```python
from build123d import *

# Parameters (mm, degrees)
SKETCH1_W               = 5.08
SKETCH1_H               = 11.684
BOSS_EXTRUDE1_DEPTH     = 8.89
SKETCH2_R               = 4.318
CUT_EXTRUDE1_DEPTH      = 8.89
BOSS_EXTRUDE4_START     = -8.89
BOSS_EXTRUDE4_DEPTH     = 8.89
BOSS_EXTRUDE5_START     = -8.89
BOSS_EXTRUDE5_DEPTH     = 8.89
SKETCH9_W               = 3.302
SKETCH9_H               = 8.128
CUT_EXTRUDE4_DEPTH      = 8.89
CUT_EXTRUDE5_REACH      = 23.984
CUT_EXTRUDE5_END_RADIUS = 4.318
SKETCH10_R              = 1.905
SKETCH11_W              = 2.413
SKETCH11_H              = 8.89
SKETCH11_W_2            = 1.778
BOSS_EXTRUDE6_DEPTH     = 17.78
CUT_EXTRUDE6_REACH      = 27.049
SKETCH12_R              = 1.905
CUT_EXTRUDE7_START      = -8.89
CUT_EXTRUDE7_DEPTH      = 8.89
FILLET3_R               = 0.635
FILLET4_R               = 1.905


with BuildPart() as part:
    # Sketch1 → Boss-Extrude1 (new body)
    with BuildSketch(Plane(origin=(0, 0, 0), x_dir=(1, 0, 0), z_dir=(0, 1, 0))):
        Rectangle(SKETCH1_W, SKETCH1_H)
    extrude(amount=BOSS_EXTRUDE1_DEPTH)

    # Sketch2 → Cut-Extrude1 (cut)
    with BuildSketch(Plane(origin=(0, 8.89, 0), x_dir=(1, 0, 0), z_dir=(0, 1, 0))):
        with Locations((-5.08, 0)):
            Circle(SKETCH2_R)
    extrude(amount=-CUT_EXTRUDE1_DEPTH, mode=Mode.SUBTRACT)

    # Sketch7 → Boss-Extrude4 (add)
    with BuildSketch(Plane.XZ.offset(BOSS_EXTRUDE4_START)):
        with BuildLine():
            Line((-2.54, 3.49192268), (-2.54, 5.842))
            ThreePointArc((-2.54, 5.842), (-11.450287592, 0), (-2.54, -5.842))
            Line((-2.54, -5.842), (-2.54, -3.49192268))
            ThreePointArc((-2.54, -3.49192268), (-9.398, 0), (-2.54, 3.49192268))
        make_face()
    extrude(amount=BOSS_EXTRUDE4_DEPTH)

    # Sketch8 → Boss-Extrude5 (add)
    with BuildSketch(Plane.XZ.offset(BOSS_EXTRUDE5_START)):
        with BuildLine():
            Line((-7.894132015, 5.715), (-16.530287592, 5.715))
            Line((-16.530287592, 5.715), (-16.530287592, -5.715))
            Line((-16.530287592, -5.715), (-7.894132015, -5.715))
            ThreePointArc((-7.894132015, -5.715), (-11.450287592, 0), (-7.894132015, 5.715))
        make_face()
    extrude(amount=BOSS_EXTRUDE5_DEPTH)

    # Sketch9 → Cut-Extrude4 (cut)
    with BuildSketch(Plane.XZ):
        with Locations((-12.339287592, 0)):
            Rectangle(SKETCH9_W, SKETCH9_H)
    extrude(amount=-CUT_EXTRUDE4_DEPTH, mode=Mode.SUBTRACT)

    # Cut-Extrude5: up to this cylinder (the profile starts outside it)
    cut_extrude5_end = Plane(origin=(-5.08, 4.445, 0), z_dir=(0, 1, 0)) * Cylinder(CUT_EXTRUDE5_END_RADIUS, 57.604, mode=Mode.PRIVATE)
    # Sketch10 → Cut-Extrude5 (cut, up to the surface)
    with BuildSketch(Plane.ZY.offset(16.530287592), mode=Mode.PRIVATE) as cut_extrude5_sk1:
        with Locations((0, 4.445)):
            Circle(SKETCH10_R)
    cut_extrude5_tool1 = extrude(cut_extrude5_sk1.sketch, amount=-CUT_EXTRUDE5_REACH, mode=Mode.PRIVATE) - cut_extrude5_end
    add(cut_extrude5_tool1.solids().sort_by_distance((-16.530288, 4.445, 0))[0], mode=Mode.SUBTRACT)

    # Sketch11 → Boss-Extrude6 (add)
    with BuildSketch(Plane(origin=(2.54, 0, 0), x_dir=(0, 0, -1), z_dir=(1, 0, 0))):
        with Locations((0, 4.445)):
            Rectangle(SKETCH11_W, SKETCH11_H)
        with Locations((4.3815, 4.445)):
            Rectangle(SKETCH11_W_2, SKETCH11_H)
        with Locations((-4.3815, 4.445)):
            Rectangle(SKETCH11_W_2, SKETCH11_H)
    extrude(amount=BOSS_EXTRUDE6_DEPTH)

    # Cut-Extrude6: up to this face of the body (flat: up to its plane)
    cut_extrude6_end = Plane(part.part.faces().sort_by_distance((11.43, 4.445, -5.2705))[0])
    # Sketch12 → Cut-Extrude6 (cut, up to the picked face)
    with BuildSketch(Plane.XY.offset(5.2705), mode=Mode.PRIVATE) as cut_extrude6_sk1:
        with Locations((13.716, 4.445)):
            Circle(SKETCH12_R)
    cut_extrude6_tool1 = split(extrude(cut_extrude6_sk1.sketch, amount=-CUT_EXTRUDE6_REACH, mode=Mode.PRIVATE), bisect_by=cut_extrude6_end, keep=Keep.BOTH, mode=Mode.PRIVATE)
    add(cut_extrude6_tool1.solids().sort_by(Axis((13.716, 4.445, 5.2705), (0, 0, -1)))[0], mode=Mode.SUBTRACT)

    # Sketch13 → Cut-Extrude7 (cut)
    with BuildSketch(Plane(origin=(0, 8.89, 0), x_dir=(1, 0, 0), z_dir=(0, 1, 0)).offset(CUT_EXTRUDE7_START)):
        with BuildLine():
            Line((11.637890342, 3.4925), (15.794109658, 3.4925))
            ThreePointArc((15.794109658, 3.4925), (13.716, 4.064), (11.637890342, 3.4925))
        make_face()
        with BuildLine():
            Line((11.637890342, -3.4925), (15.794109658, -3.4925))
            ThreePointArc((15.794109658, -3.4925), (13.716, -4.064), (11.637890342, -3.4925))
        make_face()
    extrude(amount=CUT_EXTRUDE7_DEPTH, mode=Mode.SUBTRACT)

    # Fillet3
    # the kernel refuses this fillet: 0.635 mm, written as the material it takes off along each edge
    with BuildSketch(Plane(origin=(2.54, -1.579542556, -5.842), x_dir=(-1, 0, 0), z_dir=(0, 1, 0))) as fillet3_piece_1:
        with BuildLine():
            CenterArc((0.631817023, 0.635), FILLET3_R, 185.739170477, 84.260829523)
            Line((0, 0.5715), (-0.01263634, 0.57023))
            ThreePointArc((-0.01263634, 0.57023), (-0.0127, 0.28575), (-0.0127, 0))
            Line((-0.0127, 0), (0, -0.0127))
            Line((0, -0.0127), (0.631817023, -0.0127))
            Line((0.631817023, -0.0127), (0.631817023, 0))
        make_face()
    extrude(amount=12.049085113, mode=Mode.SUBTRACT)
    with BuildSketch(Plane(origin=(2.54, -1.579542556, 5.842), x_dir=(-1, 0, 0), z_dir=(0, 1, 0))) as fillet3_piece_2:
        with BuildLine():
            CenterArc((0.631817023, -0.635), FILLET3_R, 90, 84.260829523)
            Line((0, -0.5715), (-0.01263634, -0.57023))
            ThreePointArc((-0.01263634, -0.57023), (-0.0127, -0.28575), (-0.0127, 0))
            Line((-0.0127, 0), (0, 0.0127))
            Line((0, 0.0127), (0.631817023, 0.0127))
            Line((0.631817023, 0.0127), (0.631817023, 0))
        make_face()
    extrude(amount=12.049085113, mode=Mode.SUBTRACT)

    # Fillet4
    fillet4_edges = [part.edges().sort_by_distance(p)[0] for p in [
        (-16.530287592, 4.445, 5.715),
        (-16.530287592, 4.445, -5.715),
        (20.32, 0, 0),
        (20.32, 8.89, 0),
        (20.32, 8.89, -4.3815),
        (20.32, 0, -4.3815),
        (20.32, 0, 4.3815),
        (20.32, 8.89, 4.3815),
    ]]
    fillet(fillet4_edges, radius=FILLET4_R)


solid = part.part
```
Work out the finished part from the listing and answer in its coordinate system (mm). A direction names the side the tool comes from. Round coordinates to 2 decimals unless told otherwise and drop trailing zeros. Write each loop counter-clockwise with the first axis right and the second up, starting at its lowest first coordinate (ties: lowest second). Pieces come first, ordered by that corner, then holes. Notation, with made-up numbers: (45.5, -28) - (95.5, -28) arc R17 cw to (95.5, -6) - close; hole circle Ø9 at (62.5, -35). An arc over 180 degrees is marked (long way). Return JSON: item names as keys, results as strings. Group by question number.
Q1. The part is cut by section D-D on y = 0.75. Count the separate pieces of the cut face and the enclosed holes in it, then the cut area to 3 significant figures.
Q2. For faces 1 (the flat face through (2.54, 4, 2)), 2 (the flat face through (-11, 5, -5.715)), 3 (the flat face through (0, 4, -5.842)), 4 (the cylindrical face through (14.23, 2.41, 4.03)), determine the directions among +Z, -Z, +X, -X, +Y, -Y from which every point of the face is accessible in a straight line to the end or side of a thin tool.
Q3. The mould has two halves that part along X. Classify faces 5 (the flat face through (7, 4, -3.492)), 6 (the flat face through (2.54, 4, -2)), 7 (the flat face through (-13.99, 2, 0)): released by +X, released by -X, zero draft, split by the parting line, or undercut.
Q4. The part is cut by section A-A on z = 0. Write down the section's boundary in (x, y) (3 decimals), then the cut area to 3 significant figures.
Q5. Find the intervals of material crossed by L1, parallel to Z at x = 4, y = 4.5; L2, parallel to Z at x = -11.5, y = 5 (3 decimals); L3, parallel to X at y = 7.5, z = -2.25, in increasing order.
Q6. The part is cut by section C-C on x = -5.08. Write down the section's boundary in (y, z).
Q7. The part is cut by section B-B on x = 5. Write down the section's boundary in (y, z).
Q8. Each of these flat-tipped pins is pushed along its axis until it touches: pin 1 Ø2.5 at (x, y) = (18, 2.5) entering from -Z; pin 2 Ø2.5 at (x, y) = (8.5, 6) entering from +Z; pin 3 Ø2.5 at (x, y) = (-12.5, 4) entering from -Z (3 decimals). Where does it stop, or does it pass through?
Solved:
{
 "1": {"separate pieces": "1", "enclosed holes": "2", "area": "238 mm²"},
 "2": {"face 1": "+X, +Y, -Y", "face 2": "-Z, -X, +Y, -Y", "face 3": "-Z, +X, +Y, -Y", "face 4": "+Y, -Y"},
 "3": {"face 5": "zero draft", "face 6": "released by +X", "face 7": "undercut"},
 "4": {"outline": "(-16.53, 0) - (-13.99, 0) - (-13.99, 2.54) - (-16.53, 2.54) - close; (-16.53, 6.35) - (-13.99, 6.35) - (-13.99, 8.89) - (-16.53, 8.89) - close; (-10.688, 0) - (-9.398, 0) - (-9.398, 2.54) - (-10.688, 2.54) - close; (-10.688, 6.35) - (-9.398, 6.35) - (-9.398, 8.89) - (-10.688, 8.89) - close; (-0.762, 0) - (18.415, 0) arc R1.905 ccw to (20.32, 1.905) - (20.32, 6.985) arc R1.905 ccw to (18.415, 8.89) - (-0.762, 8.89) - close; hole circle Ø3.81 at (13.716, 4.445)", "area": "194 mm²"},
 "5": {"L1": "-5.27 to -3.49, -1.21 to 1.21, 3.49 to 5.27", "L2": "-5.715 to -4.064, 4.064 to 5.715", "L3": "-16.53 to -13.99, -10.69 to -8.77, -1.39 to 2.54"},
 "6": {"outline": "(0, -6.37) - (8.89, -6.37) - (8.89, -4.32) - (0, -4.32) - close; (0, 4.32) - (8.89, 4.32) - (8.89, 6.37) - (0, 6.37) - close"},
 "7": {"outline": "(0, -5.27) - (8.89, -5.27) - (8.89, -3.49) - (0, -3.49) - close; (0, -1.21) - (8.89, -1.21) - (8.89, 1.21) - (0, 1.21) - close; (0, 3.49) - (8.89, 3.49) - (8.89, 5.27) - (0, 5.27) - close"},
 "8": {"pin 1": "z = -5.27", "pin 2": "z = 5.27", "pin 3": "z = -5.715"}
}
